Autodesk Inventor part; units mm, degrees
ref_plane "YZ Plane" through (0, 0, 0) normal (1, 0, 0) x (0, 1, 0)
ref_plane "XZ Plane" through (0, 0, 0) normal (0, 1, 0) x (-1, 0, 0)
ref_plane "XY Plane" through (0, 0, 0) normal (0, 0, 1) x (1, 0, 0)
ref_plane "Plano de trabajo1" through (0, 0, 0) normal (0, 0, 1) x (1, 0, 0)
sketch "Boceto1" plane through (0, 0, 0) normal (0, 0, 1) x (1, 0, 0)
  line L0 (-72.9949, 0) -> (-72.9949, 3)
  line L1 (-72.9949, 3) -> (-72.9949, -3)
  line L2 (-72.9949, -3) -> (-22.9949, -3)
  line L3 (-22.9949, -3) -> (-22.9949, 3)
  line L4 (-22.9949, 3) -> (-72.9949, 3)
  point P0 (0, 0)
  dimension "d0" = 3
  dimension "d1" = 6
  dimension "d2" = 50
  dimension "d3" = 90
  dimension "d4" = 6
extrude "Extrusión1" add sketch "Boceto1" along normal blind 115
sketch "Boceto2" plane through (-72.9949, 3, 0) normal (0, 1, 0) x (1, 0, 0)
  line L0 (0, 0) -> (0, -115)
  line L1 (0, 0) -> (3, 0)
  line L2 (3, 0) -> (3, -20.4)
  line L3 (3, -20.4) -> (0, -20.4)
  line L4 (0, -20.4) -> (0, 0)
  point P0 (72.9949, 0)
  dimension "d7" = 3
  dimension "d8" = 20.4
extrude "Extrusión2" cut sketch "Boceto2" against normal blind 6
sketch "Boceto3" plane through (-72.9949, 3, 115) normal (0, 1, 0) x (1, 0, 0)
  line L0 (3, 115) -> (50, 115)
  line L1 (3, 115) -> (5, 115)
  line L2 (5, 115) -> (5, 94.6)
  line L3 (5, 94.6) -> (3, 94.6)
  line L4 (3, 94.6) -> (3, 115)
  point P0 (72.9949, 115)
  dimension "d11" = 2
  dimension "d12" = 20.4
extrude "Extrusión3" add sketch "Boceto3" along normal blind 17
sketch "Boceto5" plane through (-72.9949, -3, 115) normal (0, -1, 0) x (1, 0, 0)
  line L0 (3, -94.6) -> (0, -94.6)
  line L1 (3, -94.6) -> (5, -94.6)
  line L2 (5, -94.6) -> (5, -115)
  line L3 (5, -115) -> (3, -115)
  line L4 (3, -115) -> (3, -94.6)
  point P0 (72.9949, -115)
  dimension "d15" = 2
  dimension "d16" = 20.4
extrude "Extrusión4" add sketch "Boceto5" along normal blind 17
fillet "Empalme1" radius 2 2 edges at (-68.9949, -20, 20.4) (-68.9949, 20, 20.4)
sketch "Boceto6" plane through (-69.9949, -20, 0) normal (-1, 0, 0) x (0, 0, 1)
  circle A0 centre (10.1353, 9.969) radius 1.7
  circle A1 centre (10.1353, 30.0745) radius 1.7
  point P0 (0, 20)
  dimension "d20" = 3.4
  dimension "d21" = 3.4
extrude "Extrusión5" cut sketch "Boceto6" against normal blind 2
sketch "Boceto7" plane through (-72.9949, -3, 115) normal (0, -1, 0) x (1, 0, 0)
  line L0 (0, 0) -> (2, 0)
  line L1 (2, 0) -> (2, -20)
  line L2 (2, -20) -> (0, -20)
  line L3 (0, -20) -> (0, 0)
  point P0 (72.9949, -115)
  dimension "d24" = 2
  dimension "d25" = 20
extrude "Extrusión6" add sketch "Boceto7" along normal blind 20
sketch "Boceto8" plane through (-72.9949, 3, 115) normal (0, 1, 0) x (1, 0, 0)
  line L0 (2, 20) -> (2, 0)
  line L1 (0, 0) -> (2, 0)
  line L2 (2, 0) -> (2, 20)
  line L3 (2, 20) -> (0, 20)
  line L4 (0, 20) -> (0, 0)
  point P0 (72.9949, 115)
  dimension "d28" = 2
  dimension "d29" = 20
extrude "Extrusión7" add sketch "Boceto8" along normal blind 20
sketch "Boceto9" plane through (-72.9949, -3, 20.4) normal (-1, 0, 0) x (0, 0, 1)
  circle A0 centre (85.3122, 16) radius 1.7
  circle A1 centre (85.3122, -10.078) radius 1.7
  point P0 (-20.4, 3)
  dimension "d32" = 3.4
  dimension "d33" = 3.4
extrude "Extrusión8" cut sketch "Boceto9" against normal blind 20
fillet "Empalme2" radius 2 2 edges at (-71.9949, 23, 95) (-71.9949, -23, 95)
sketch "Boceto10" plane through (-22.9949, 3, 115) normal (0, 1, 0) x (1, 0, 0)
  line L0 (0, 115) -> (0, 0)
  line L1 (0, 115) -> (0, 57.5)
  line L2 (0, 57.5) -> (0, 86.25)
  line L3 (0, 57.5) -> (28.75, 57.5) construction
  line L4 (0, 86.25) -> (0, 28.75)
  line L5 (-50, 94.6) -> (-50, 20)
  line L6 (-50, 57.3) -> (-30, 57.3)
  line L7 (-50, 57.3) -> (-30, 57.3) construction
  line L8 (0, 86.25) -> (0, 28.75)
  arc A0 (0, 86.25) -> (0, 28.75) centre (-1.2246, 57.5) ccw
  point P0 (22.9949, 115)
  dimension "d37" = 57.5
  dimension "d39" = 28.75
  dimension "d40" = 90
  dimension "d41" = 57.5
  dimension "d42" = 0
  dimension "d43" = 20
  dimension "d44" = 0
extrude "Extrusión9" cut sketch "Boceto10" against normal blind 20
fillet "Empalme3" radius 5 2 edges at (-22.9949, 0, 86.25) (-22.9949, 0, 28.75)
fillet "Empalme4" radius 3 5 edges at (-22.9949, -3, 11.9678) (-24.267, -3, 87.7323) (-24.267, -3, 27.2677) (-52.9955, -3, 57.5) (-22.9949, -3, 103.0322)
properties part number "SoporteAmbu"
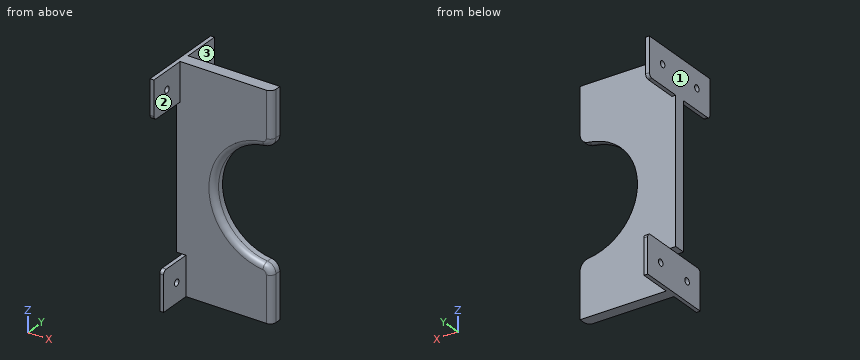
Geometry: final body of the model. Coordinates: model frame, mm. Face numbers are marked on the shaded views. A direction names the side the tool comes from. Round coordinates to 2 decimals unless told otherwise and drop trailing zeros. Order: outer loops, then holes, each group sorted by start corner. A loop starts at its lowest first (then second) coordinate and runs counter-clockwise, first axis right, second up.
Q1. Material intervals for probe 1 along Z at (x, y) = (-69, -10); probe 2 along X at (y, z) = (-14, 6); probe 3 along Y at (x, z) = (-65.5, 43), sorted ascending.
Result sheet:
probe 1: z = 0 to 8.44, 11.84 to 20.4
probe 2: x = -69.99 to -67.99
probe 3: y = -3 to 3
Q2. Access query for the marked faces 1, 2 and 3. Directions: +Z, -Z, +X, -X, +Y, -Y. A direction counts if a zero-diameter tool reaches every point of the face in a straight line with its end or side. Return the directions, or none.
Result sheet:
face 1: +Z, -Z, -X, +Y, -Y
face 2: +Z, -Z, +X, -Y
face 3: +Z, -Z, +X, +Y
Q3. Pin query (flat end, axial travel): pin 1 (1.6 mm diameter, centred on x = -69, z = 5, fed in from +Y); pin 2 (8.5 mm diameter, centred on y = 13, z = 5.5, fed in from +X); pin 3 (2 mm diameter, centred on y = 14.5, z = 18, fed in from -X). Return the tip coordinate at first contact, or that it passes through.
Result sheet:
pin 1: stops at y = 20
pin 2: stops at x = -67.99
pin 3: stops at x = -69.99
Q4. Section A-A, the plane y = 13. Output: boundary loops of the cut face in (x, z), and give its area (3 significant figures).
Result sheet:
outline: (-72.99, 95) - (-70.99, 95) - (-70.99, 104.01) - (-72.99, 104.01) - close; (-72.99, 107.41) - (-70.99, 107.41) - (-70.99, 115) - (-72.99, 115) - close; (-69.99, 0) - (-67.99, 0) - (-67.99, 20.4) - (-69.99, 20.4) - close
area: 74.0 mm2
Q5. Section B-B, the plane y = 5.5. Output: boundary loops of the cut face in (x, z).
Result sheet:
outline: (-72.99, 95) - (-70.99, 95) - (-70.99, 115) - (-72.99, 115) - close; (-69.99, 0) - (-67.99, 0) - (-67.99, 20.4) - (-69.99, 20.4) - close
Q6. Section C-C, the plane x = -65. Output: boundary loops of the cut face in (y, z).
Result sheet:
outline: (-3, 0) - (3, 0) - (3, 115) - (-3, 115) - close
